Work out the finished part from the listing and answer in its coordinate system (mm). Face numbers are marked on the shaded views. Round coordinates to 2 decimals unless told otherwise and drop trailing zeros. Order: outer loops, then holes, each group sorted by start corner. A loop starts at its lowest first (then second) coordinate and runs counter-clockwise, first axis right, second up. Notation, with made-up numbers: (41, -39.5) -> (48, -39.5) arc R23 cw to (48, -3.5) -> close; hole circle Ø1 at (57.5, 57). An arc over 180 degrees is marked (long way). Use one line per item in the form item = value.
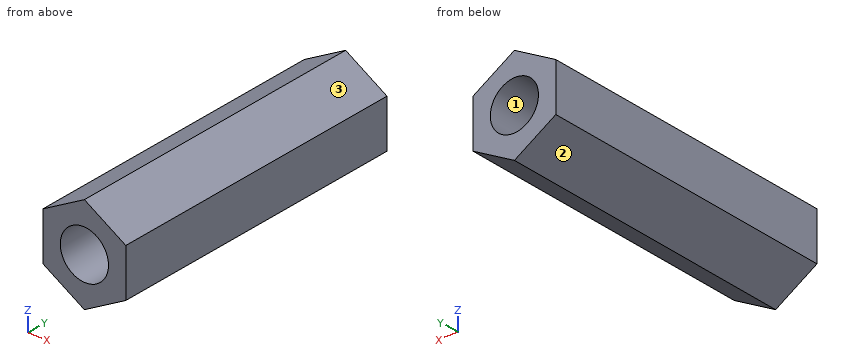
Autodesk Inventor part; units mm, degrees
ref_plane "YZ Plane" through (0, 0, 0) normal (1, 0, 0) x (0, 1, 0)
ref_plane "XZ Plane" through (0, 0, 0) normal (0, 1, 0) x (-1, 0, 0)
ref_plane "XY Plane" through (0, 0, 0) normal (0, 0, 1) x (1, 0, 0)
sketch "Sketch1" plane through (0, 0, 0) normal (0, 1, 0) x (-1, 0, 0)
  line L0 (0, -7.3323) -> (-6.35, -3.6662)
  line L1 (-6.35, -3.6662) -> (-6.35, 3.6662)
  line L2 (-6.35, 3.6662) -> (0, 7.3323)
  line L3 (0, 7.3323) -> (6.35, 3.6662)
  line L4 (6.35, 3.6662) -> (6.35, -3.6662)
  line L5 (6.35, -3.6662) -> (0, -7.3323)
  point P0 (0, 0)
  point P1 (0, 0)
  dimension "d0" = 12.7
extrude "Extrusion1" add sketch "Sketch1" along normal blind 45.5422
sketch "Sketch2" plane through (0, 45.5422, 0) normal (0, 1, 0) x (1, 0, 0)
  circle A0 centre (0, 0) radius 3.6957
  dimension "d3" = 7.3914
extrude "Extrusion2" cut sketch "Sketch2" against normal blind 45.5422
thread "Thread1"
properties part number "hexshaft_gearbox2"
Item 1: Consider line 1 along Z through (x, y) = (0, 15.5); line 2 along X through (y, z) = (43, -0.5); line 3 along X through (y, z) = (8, -1.75). Determine where each line is inside the solid, lowest interval first.
Findings:
line_1 = -7.33 to -3.7, 3.7 to 7.33
line_2 = -6.35 to -3.66, 3.66 to 6.35
line_3 = -6.35 to -3.26, 3.26 to 6.35
Item 2: The part is cut by section D-D, the plane x = 4.25. Give the vertices of the cut face in (y, z), and give its area (3 significant figures).
Findings:
outline = (0, -4.88) -> (45.54, -4.88) -> (45.54, 4.88) -> (0, 4.88) -> close
area = 444 mm^2
Item 3: The part is cut by section A-A, the plane y = 5. Give the vertices of the cut face in (x, z).
Findings:
outline = (-6.35, -3.67) -> (0, -7.33) -> (6.35, -3.67) -> (6.35, 3.67) -> (0, 7.33) -> (-6.35, 3.67) -> close; hole circle Ø7.39 at (0, 0)
Item 4: Flat-ended cylindrical pins translate along their axes: P1, Ø5, axis at x = 1, y = 33.5, coming from the -Z side; P2, Ø4.5, axis at x = 0, z = 0, coming from the -Y side. Find the tip coordinate at first contact, or state that the pin passes through.
Findings:
P1 = -7.33
P2 = through
Item 5: The part is cut by section B-B, the plane z = 0. Give the vertices of the cut face in (x, y), and give its area (3 significant figures).
Findings:
outline = (-6.35, 0) -> (-3.7, 0) -> (-3.7, 45.54) -> (-6.35, 45.54) -> close; (3.7, 0) -> (6.35, 0) -> (6.35, 45.54) -> (3.7, 45.54) -> close
area = 242 mm^2
Item 6: The part is cut by section C-C, the plane x = -2.5. Give the vertices of the cut face in (y, z).
Findings:
outline = (0, -5.89) -> (45.54, -5.89) -> (45.54, -2.72) -> (0, -2.72) -> close; (0, 2.72) -> (45.54, 2.72) -> (45.54, 5.89) -> (0, 5.89) -> close
Item 7: Determine the mould class of the marked faces 1, 2 and 3 for opening direction X: released by +X, released by -X, zero draft, split by the parting line, or undercut.
Findings:
face_1 = undercut
face_2 = released by -X
face_3 = released by +X
